from build123d import *

# Parameters (mm, degrees)
F1_DEPTH       = 19.05
F2_R           = 0.79999
F4_D           = 3.4
F4_CSINK_D     = 6.8
F4_CSINK_ANGLE = 90


# Not quite as in the source:
# - a fillet or chamfer is up to 0.001 mm smaller than in the source, because OpenCascade refuses the exact size


with BuildPart() as f1:
    # F0 (on Top) → F1 (new body)
    with BuildSketch(Plane.XY):
        with BuildLine():
            ThreePointArc((18.475572213, 3.2577418652), (11.1789988923, -9.3802938474), (0, 0))
            Line((0, 0), (0, 18.25))
            ThreePointArc((0, 18.25), (-0.2343145751, 18.8156854249), (-0.8, 19.05))
            ThreePointArc((-0.8, 19.05), (-1.3656854249, 18.8156854249), (-1.6, 18.25))
            Line((-1.6, 18.25), (-1.6, 0))
            ThreePointArc((-1.6, 0), (11.4568359765, -10.9559862523), (19.9790804062, 3.8049740945))
            Line((19.9790804062, 3.8049740945), (18.475572213, 3.2577418652))
        make_face()
    extrude(amount=F1_DEPTH)

    # F2 (radius 0.8 in the source; OpenCascade refuses exactly that, so slightly less here)
    f2_edges = [f1.edges().sort_by_distance(p)[0] for p in [
        (19.97908, 3.804974, 9.525),
        (18.475572, 3.257742, 9.525),
    ]]
    fillet(f2_edges, radius=F2_R)

    # F4 (through all)
    with Locations(Plane.YZ):
        with Locations((9.125, 9.525)):
            CounterSinkHole(F4_D / 2, F4_CSINK_D / 2, counter_sink_angle=F4_CSINK_ANGLE)


solid = f1.part
Geometry: final body of the model. Coordinates: model frame, mm. A direction names the side the tool comes from. Round coordinates to 2 decimals unless told otherwise and drop trailing zeros. Write each loop counter-clockwise with the first axis right and the second up, starting at its lowest first coordinate (ties: lowest second). Pieces come first, ordered by that corner, then holes. Notation, with made-up numbers: M 30,22.5 L 44,22.5 A24 cw 44,46.5 Z; hole C -4,-9.5 d3. An arc over 180 degrees is marked long. Write item = value, one per line.
Item 1: Material intervals for line 1 along X through (y, z) = (2, 4.75); line 2 along X through (y, z) = (13, 3.75); line 3 along Y through (x, z) = (9.5, 5.75), sorted ascending. Write a range as [from, to].
Findings:
line_1 = [-1.6, 0], [18.84, 20.47]
line_2 = [-1.6, 0]
line_3 = [-11.12, -9.52]
Item 2: Section query C-C on x = 13.5. Return loops of the section in (y, z), then the cut area to 3 significant figures.
Findings:
outline = M -10.39,0 L -8.66,0 L -8.66,19.05 L -10.39,19.05 Z
area = 33.0 mm^2
Item 3: Section query A-A on y = -3.5. Return loops of the section in (x, z).
Findings:
outline = M -1.04,0 L 0.67,0 L 0.67,19.05 L -1.04,19.05 Z; M 18.38,0 L 20.09,0 L 20.09,19.05 L 18.38,19.05 Z
Item 4: Access query for faces 1 (the face through (1, -5, 19.05)), 2 (the face through (0, 5, 9)). Directions: +Z, -Z, +X, -X, +Y, -Y. A direction counts if a zero-diameter tool reaches every point of the face in a straight line with its end or side. Return the directions, or none.
Findings:
face_1 = +Z, +X, -X, +Y, -Y
face_2 = +Z, -Z, +Y
Item 5: Section query D-D on x = 4.25. Return loops of the section in (y, z), then the cut area to 3 significant figures.
Findings:
outline = M -9.79,0 L -7.93,0 L -7.93,19.05 L -9.79,19.05 Z
area = 35.5 mm^2
Item 6: Pin query (flat end, axial travel): P1, Ø1, axis at x = 18.5, z = 13.5, coming from the -Y side; P2, Ø3, axis at y = 13, z = 9, coming from the +X side; P3, Ø1, axis at x = 18.5, y = 2, coming from the -Z side. Return the tip coordinate at first contact, or that it passes through.
Findings:
P1 = -7.21
P2 = 0
P3 = 0
Item 7: Pull-direction query (X, two-part tool) for faces 3 (the face through (1, -5, 0)), 4 (the face through (10.767, -11.055, 9.392)), 5 (the face through (18.76, 3.13, 9.66)); classes: pulls with the +X half, pulls with the -X half, needs draft (parallel to the pull), parting line crosses it, or undercut.
Findings:
face_3 = needs draft
face_4 = parting line crosses it
face_5 = undercut
